from build123d import *

# Parameters (mm, degrees)
SKETCH005_R   = 2
SKETCH005_R_2 = 2.65
PAD_DEPTH     = 4
FILLET_R      = 7
FILLET001_R   = 20
FILLET002_R   = 6
FILLET003_R   = 10
FILLET004_R   = 1
FILLET005_R   = 0.5
FILLET006_R   = 0.5


with BuildPart() as part:
    # Sketch005 → Pad (new body)
    with BuildSketch(Plane.XY.offset(-3)):
        Polygon((-33, 10), (-27, 10), (-27, 1), (-33, 1), (-33, -1), (-27, -1), (-27, -10), (13, -10), (13, -1), (19, -1), (19, 1), (13, 1), (13, 10), (20, 10), (47, 0.7), (47, -8.030345), (28, -19), (-40, -19), (-50, -13.226497), (-50, -6), align=None)
        with Locations((-31.5, 5)):
            Circle(SKETCH005_R, mode=Mode.SUBTRACT)
        with Locations((-31.5, -5)):
            Circle(SKETCH005_R, mode=Mode.SUBTRACT)
        with Locations((17.5, 5)):
            Circle(SKETCH005_R, mode=Mode.SUBTRACT)
        with Locations((17.5, -5)):
            Circle(SKETCH005_R, mode=Mode.SUBTRACT)
        with Locations((40.5, -5)):
            Circle(SKETCH005_R_2, mode=Mode.SUBTRACT)
        with Locations((-44.5, -10)):
            Circle(SKETCH005_R_2, mode=Mode.SUBTRACT)
    extrude(amount=PAD_DEPTH)

    # Fillet
    fillet_edges = [part.edges().sort_by_distance(p)[0] for p in [
        (-50, -13.226497, -1),
        (-50, -6, -1),
    ]]
    fillet(fillet_edges, radius=FILLET_R)

    # Fillet001
    fillet001_edges = [part.edges().sort_by_distance(p)[0] for p in [
        (-40, -19, -1),
        (28, -19, -1),
    ]]
    fillet(fillet001_edges, radius=FILLET001_R)

    # Fillet002
    fillet002_edges = [part.edges().sort_by_distance(p)[0] for p in [
        (47, -8.030345, -1),
        (47, 0.7, -1),
    ]]
    fillet(fillet002_edges, radius=FILLET002_R)

    # Fillet003
    fillet003_edges = [part.edges().sort_by_distance(p)[0] for p in [
        (-33, 10, -1),
        (20, 10, -1),
    ]]
    fillet(fillet003_edges, radius=FILLET003_R)

    # Fillet004
    fillet004_edges = [part.edges().sort_by_distance(p)[0] for p in [
        (13, 10, -1),
        (-27, 10, -1),
    ]]
    fillet(fillet004_edges, radius=FILLET004_R)

    # Fillet005
    fillet005_edges = [part.edges().sort_by_distance(p)[0] for p in [
        (13, -10, -1),
        (-27, -10, -1),
    ]]
    fillet(fillet005_edges, radius=FILLET005_R)

    # Fillet006
    fillet006_edges = [part.edges().sort_by_distance(p)[0] for p in [
        (-27, -1, -1),
        (-27, 1, -1),
        (13, -1, -1),
        (13, 1, -1),
    ]]
    fillet(fillet006_edges, radius=FILLET006_R)


solid = part.part
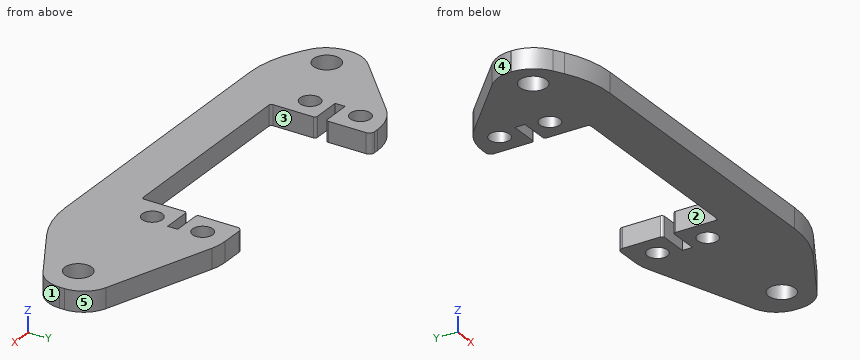
Build history of the part. All positions in model axes, mm. Face numbers are marked on the shaded views. A direction names the side the tool comes from. Give positions to 0.01 mm unless a question says otherwise; leave off trailing zeros. Loops run counter-clockwise (first coordinate to the right, second up) from the corner with the lowest first, then second, coordinate; pieces in that order, holes last. Notation, with made-up numbers: (74, 8.5) -> (132, 8.5) arc R30 ccw to (132, 46.5) -> close; hole circle Ø4 at (71, 63). An arc over 180 degrees is marked (long way). Answer in a Markdown table with one row per item.
Item 1: Mould opens along X. For the marked faces 3, 4 and 5 say: pulls with the +X half, pulls with the -X half, needs draft (parallel to the pull), parting line crosses it, or undercut.
Findings below:
| item | result |
|---|---|
| face 3 | undercut |
| face 4 | pulls with the -X half |
| face 5 | pulls with the +X half |
Item 2: Slice it at B-B on x = 17.5. Write the cut outline in (y, z), plus the area to 3 significant figures.
Findings below:
| item | result |
|---|---|
| outline | (-19, -3) -> (-7, -3) -> (-7, 1) -> (-19, 1) -> close; (-3, -3) -> (-1, -3) -> (-1, 1) -> (-3, 1) -> close; (1, -3) -> (3, -3) -> (3, 1) -> (1, 1) -> close; (7, -3) -> (10, -3) -> (10, 1) -> (7, 1) -> close |
| area | 76.0 mm² |
Item 3: Slice it at C-C on z = -0.75. Give the number of separate pieces and of enclosed holes in the cut face, plus the area to 3 significant figures.
Findings below:
| item | result |
|---|---|
| separate pieces | 1 |
| enclosed holes | 6 |
| area | 1,480 mm² |
Item 4: Slice it at D-D on x = -9. Write the cut outline in (y, z), plus the area to 3 significant figures.
Findings below:
| item | result |
|---|---|
| outline | (-19, -3) -> (-10, -3) -> (-10, 1) -> (-19, 1) -> close |
| area | 36.0 mm² |
Item 5: Probe line 1 along Y through (x, z) = (17.5, -0.6); line 2 along X through (y, z) = (-6, -1.6); line 3 along Y through (x, z) = (16.5, -0.75). List the from-to ranges inside material, lowest first. Write a range as [from, to].
Findings below:
| item | result |
|---|---|
| line 1 | y = [-19, -7], [-3, -1], [1, 3], [7, 10] |
| line 2 | x = [-49.31, -33.23], [-29.77, -27], [13, 15.77], [19.23, 38.05], [42.95, 46.83] |
| line 3 | y = [-19, -6.73], [-3.27, -1], [1, 3.27], [6.73, 10] |
Item 6: Flat gauge pins, fed straight in: P1, Ø2, axis at x = -15, z = -0.5, coming from the +Y side; P2, Ø1.2, axis at y = 3.5, z = -0.5, coming from the -X side; P3, Ø0.6, axis at y = -0.5, z = 0, coming from the +X side. Where does each tip first touch, or does it go through?
Findings below:
| item | result |
|---|---|
| P1 | stops at y = -10 |
| P2 | stops at x = -40.54 |
| P3 | stops at x = 46.32 |
Item 7: Tool access for the marked faces 1 and 2: list every direction of +Z, -Z, +X, -X, +Y, -Y with a clear straight run to the whole face (end or side of a thin tool).
Findings below:
| item | result |
|---|---|
| face 1 | +Z, -Z, +X, -Y |
| face 2 | +Z, -Z, +Y |
Item 8: Slice it at A-A on x = 40.5. Write the cut outline in (y, z), plus the area to 3 significant figures.
Findings below:
| item | result |
|---|---|
| outline | (-11.78, -3) -> (-7.65, -3) -> (-7.65, 1) -> (-11.78, 1) -> close; (-2.35, -3) -> (2.94, -3) -> (2.94, 1) -> (-2.35, 1) -> close |
| area | 37.7 mm² |
